from build123d import *

# Parameters (mm, degrees)
SKETCH1_W           = 50.8
SKETCH1_H           = 121.92
BOSS_EXTRUDE1_DEPTH = 3.2
CUT_EXTRUDE1_DEPTH  = 122.92
BOSS_EXTRUDE2_DEPTH = 121.92
SKETCH5_W           = 50.8
SKETCH5_H           = 2
BOSS_EXTRUDE3_DEPTH = 4
FILLET1_R           = 2.54


with BuildPart() as part:
    # Sketch1 → Boss-Extrude1 (new body)
    with BuildSketch(Plane.XY):
        with Locations((28.39261314, -60.96)):
            Rectangle(SKETCH1_W, SKETCH1_H)
    extrude(amount=-BOSS_EXTRUDE1_DEPTH)

    # Sketch2 → Cut-Extrude1 (cut, through all)
    with BuildSketch(Plane.XZ.offset(121.92)):
        Polygon((53.79261314, 0), (53.79261314, -3.2), (48.250050556, -3.2), align=None)
    extrude(amount=-CUT_EXTRUDE1_DEPTH, mode=Mode.SUBTRACT)

    # Sketch4 → Boss-Extrude2 (add)
    with BuildSketch(Plane.XZ.offset(121.92)):
        Polygon((2.99261314, 0), (2.99261314, -3.2), (-2.549949444, -3.2), align=None)
    extrude(amount=-BOSS_EXTRUDE2_DEPTH)

    # Sketch5 → Boss-Extrude3 (add)
    with BuildSketch(Plane.XY):
        with Locations((28.39261314, -8.96)):
            Rectangle(SKETCH5_W, SKETCH5_H)
        with Locations((28.39261314, -112.96)):
            Rectangle(SKETCH5_W, SKETCH5_H)
    extrude(amount=BOSS_EXTRUDE3_DEPTH)

    # Fillet1
    fillet1_edges = [part.edges().sort_by_distance(p)[0] for p in [
        (28.39261314, -7.96, 0),
        (28.39261314, -113.96, 0),
    ]]
    fillet(fillet1_edges, radius=FILLET1_R)


solid = part.part
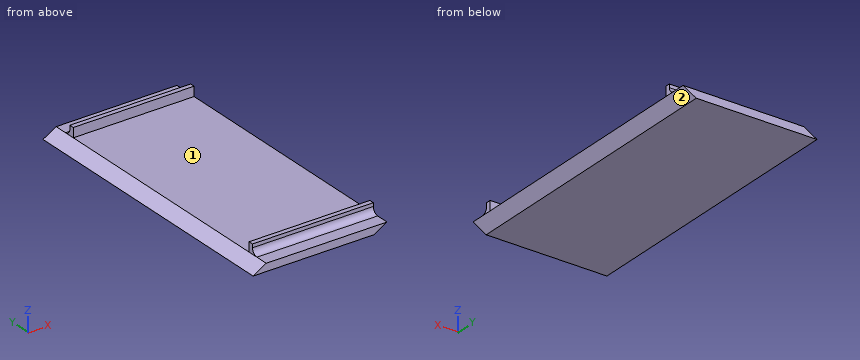
Geometry check sheet. Reference: the model listing, model coordinates, mm. Face numbers are marked on the shaded views. Coordinates: 2 decimals unless noted, no trailing zeros. Order: outer loops, then holes, each group sorted by start corner. A loop starts at its lowest first (then second) coordinate and runs counter-clockwise, first axis right, second up. Notation, with made-up numbers: (59.25, 68) -> (71.25, 68) arc R26 ccw to (71.25, 103) -> close; hole circle Ø3 at (-8, -24). An arc over 180 degrees is marked (long way). Use a Markdown table: item, result. Add a question column.
1. Cross-section at C-C (y = -31). Enter the section's corners in (x, z), and give its area (3 significant figures).
2. Cross-section at D-D (x = 49.5). Enter the section's corners in (y, z), and give its area (3 significant figures).
3. Mould release check, pull along Y, two halves, no side actions. Record for the marked faces 1 and 2: pulls with the +Y half, pulls with the -Y half, needs draft (parallel to the pull), parting line crosses it, or undercut.
4. Material ranges on L1, parallel to Y at x = 17, z = 2.75; L2, parallel to Y at x = 11, z = 2.25; L3, parallel to Z at x = 15, y = -95.5, recorded low to high.
5. Cross-section at A-A (x = 18). Enter the section's corners in (y, z).
6. Go/stop test with flat-tipped pins: pin 1 Ø3 at (x, z) = (18.5, 1) entering from -Y; pin 2 Ø3 at (x, z) = (22.5, 2) entering from +Y; pin 3 Ø6 at (x, y) = (24, -118.5) entering from +Z; pin 4 Ø4.5 at (x, y) = (24, -2) entering from +Z. Record where each tip stops, or that it passes through.
7. Cross-section at B-B (z = -1.25). Enter the section's corners in (x, y), and give its area (3 significant figures).
Filled sheet:
| question | item | result |
|---|---|---|
| 1 | outline | (-2.55, -3.2) -> (48.25, -3.2) -> (53.79, 0) -> (2.99, 0) -> close |
| 1 | area | 163 mm2 |
| 2 | outline | (-121.92, -2.48) -> (0, -2.48) -> (0, 0) -> (-5.42, 0) arc R2.54 cw to (-7.96, 2.54) -> (-7.96, 4) -> (-9.96, 4) -> (-9.96, 0) -> (-111.96, 0) -> (-111.96, 4) -> (-113.96, 4) -> (-113.96, 2.54) arc R2.54 cw to (-116.5, 0) -> (-121.92, 0) -> close |
| 2 | area | 321 mm2 |
| 3 | face 1 | undercut |
| 3 | face 2 | needs draft |
| 4 | L1 | -113.96 to -111.96, -9.96 to -7.96 |
| 4 | L2 | -113.98 to -111.96, -9.96 to -7.94 |
| 4 | L3 | -3.2 to 0 |
| 5 | outline | (-121.92, -3.2) -> (0, -3.2) -> (0, 0) -> (-5.42, 0) arc R2.54 cw to (-7.96, 2.54) -> (-7.96, 4) -> (-9.96, 4) -> (-9.96, 0) -> (-111.96, 0) -> (-111.96, 4) -> (-113.96, 4) -> (-113.96, 2.54) arc R2.54 cw to (-116.5, 0) -> (-121.92, 0) -> close |
| 6 | pin 1 | y = -121.92 |
| 6 | pin 2 | y = -6.93 |
| 6 | pin 3 | z = 0.21 |
| 6 | pin 4 | z = 0 |
| 7 | outline | (0.83, -121.92) -> (51.63, -121.92) -> (51.63, 0) -> (0.83, 0) -> close |
| 7 | area | 6,190 mm2 |
